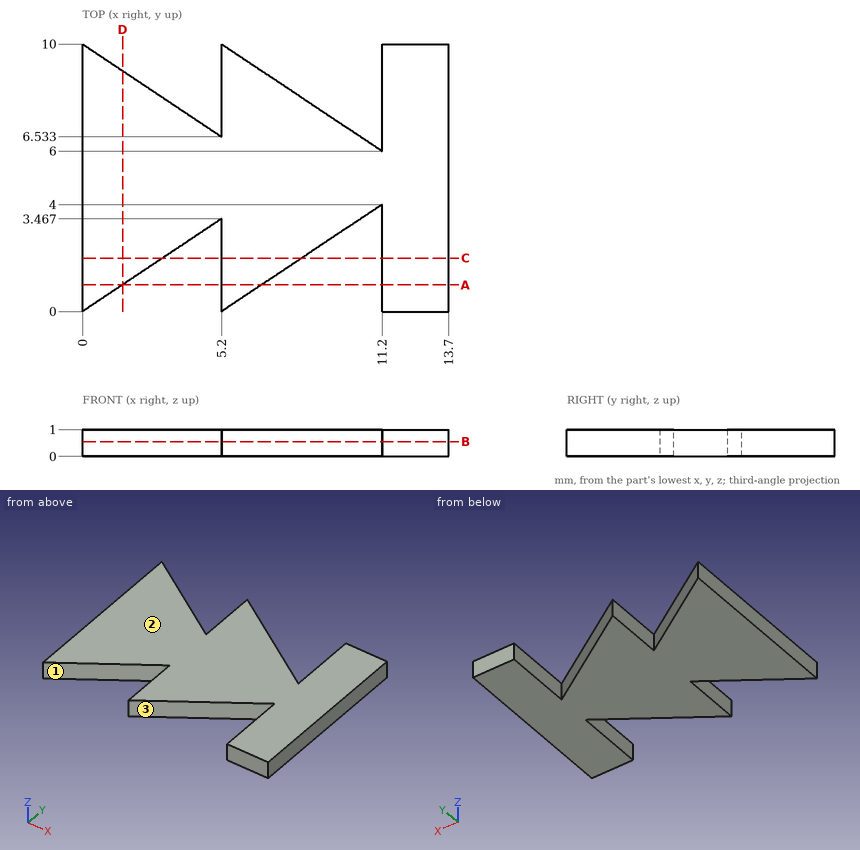
Input: dimensioned drawing with shaded views. Units: mm. Origin: part minimum x, y, z. Coordinates: 2 decimals unless noted, no trailing zeros. Write each loop counter-clockwise with the first axis right and the second up, starting at its lowest first coordinate (ties: lowest second). Pieces come first, ordered by that corner, then holes. Notation, with made-up numbers: (-16.75, -7.5) -> (31.25, -7.5) arc R25 cw to (31.25, 31.5) -> close; hole circle Ø9 at (44.25, 60). An arc over 180 degrees is marked (long way). Return JSON: item names as keys, results as strings. Group by question number.
1) Section query D-D, the plane x = 1.5. Return loops of the section in (y, z).
2) Ray query, line 1 along X through (y, z) = (8, 0.65); line 2 along X through (y, z) = (2.25, 0.45) (1 decimal); line 3 along X through (y, z) = (6.25, 0.95) (1 decimal). Return the intervals inside material, ascending.
3) Section query B-B, the plane z = 0.55. Return loops of the section in (x, y).
4) Section query C-C, the plane y = 2. Return loops of the section in (x, z).
5) Section query A-A, the plane y = 1. Return loops of the section in (x, z).
6) Mould query, pull axis X, two halves, no side actions, for the marked faces 1, 2 and 3. Classes: +X half, -X half, draft (parallel to the pull), parting line (faces both ways), or undercut.
From the geometry:
{
 "1": {"outline": "(1, 0) -> (9, 0) -> (9, 1) -> (1, 1) -> close"},
 "2": {"line 1": "0 to 3, 5.2 to 8.2, 11.2 to 13.7", "line 2": "0 to 3.4, 5.2 to 8.6, 11.2 to 13.7", "line 3": "0 to 10.8, 11.2 to 13.7"},
 "3": {"outline": "(0, 0) -> (5.2, 3.47) -> (5.2, 0) -> (11.2, 4) -> (11.2, 0) -> (13.7, 0) -> (13.7, 10) -> (11.2, 10) -> (11.2, 6) -> (5.2, 10) -> (5.2, 6.53) -> (0, 10) -> close"},
 "4": {"outline": "(0, 0) -> (3, 0) -> (3, 1) -> (0, 1) -> close; (5.2, 0) -> (8.2, 0) -> (8.2, 1) -> (5.2, 1) -> close; (11.2, 0) -> (13.7, 0) -> (13.7, 1) -> (11.2, 1) -> close"},
 "5": {"outline": "(0, 0) -> (1.5, 0) -> (1.5, 1) -> (0, 1) -> close; (5.2, 0) -> (6.7, 0) -> (6.7, 1) -> (5.2, 1) -> close; (11.2, 0) -> (13.7, 0) -> (13.7, 1) -> (11.2, 1) -> close"},
 "6": {"face 1": "undercut", "face 2": "draft", "face 3": "undercut"}
}
